Read the model definition and answer for the solid it produces. Units are mm, in the model's axes. A direction names the side the tool comes from. Coordinates: 2 decimals unless noted, no trailing zeros. Order: outer loops, then holes, each group sorted by start corner. A loop starts at its lowest first (then second) coordinate and runs counter-clockwise, first axis right, second up. Notation, with made-up numbers: (74.5, -27.5) -> (130.5, -27.5) arc R33 ccw to (130.5, 1.5) -> close; hole circle Ø5 at (60, 25). An arc over 180 degrees is marked (long way). Return JSON: item names as keys, results as strings. Group by question number.
```python
from build123d import *

# Parameters (mm, degrees)
F1_DEPTH  = 460
F3_D      = 6.5
F5_D      = 6.5
F7_D      = 6.5
F9_D      = 10.5
F9_DEPTH  = 3
F9_TIP    = 3.1545182499
F11_D     = 10.5
F11_DEPTH = 3
F11_TIP   = 3.1545182499
F13_D     = 10.5
F13_DEPTH = 3
F13_TIP   = 3.1545182499


with BuildPart() as f1:
    # F0 (on Front) → F1 (new body)
    with BuildSketch(Plane.XZ):
        Polygon((0, 10), (0, 0), (30, 0), (30, 5), (20, 5), (20, 10), align=None)
    extrude(amount=-F1_DEPTH)

    # F3 (through all)
    with Locations(Plane(origin=(0, 0, 0), x_dir=(1, 0, 0), z_dir=(0, 0, -1))):
        with Locations((10, -440)):
            Hole(F3_D / 2)

    # F5 (through all)
    with Locations(Plane(origin=(0, 0, 0), x_dir=(1, 0, 0), z_dir=(0, 0, -1))):
        with Locations((10, -230)):
            Hole(F5_D / 2)

    # F7 (through all)
    with Locations(Plane(origin=(0, 0, 0), x_dir=(1, 0, 0), z_dir=(0, 0, -1))):
        with Locations((10, -20)):
            Hole(F7_D / 2)

    # F9
    with Locations(Plane(origin=(0, 0, 0), x_dir=(1, 0, 0), z_dir=(0, 0, -1))):
        with Locations((10, -440)):
            Hole(F9_D / 2, depth=F9_DEPTH)
            with Locations((0, 0, -(F9_DEPTH + F9_TIP / 2))):  # 118° drill point
                Cone(0, F9_D / 2, F9_TIP, mode=Mode.SUBTRACT)

    # F11
    with Locations(Plane(origin=(0, 0, 0), x_dir=(1, 0, 0), z_dir=(0, 0, -1))):
        with Locations((10, -230)):
            Hole(F11_D / 2, depth=F11_DEPTH)
            with Locations((0, 0, -(F11_DEPTH + F11_TIP / 2))):  # 118° drill point
                Cone(0, F11_D / 2, F11_TIP, mode=Mode.SUBTRACT)

    # F13
    with Locations(Plane(origin=(0, 0, 0), x_dir=(1, 0, 0), z_dir=(0, 0, -1))):
        with Locations((10, -20)):
            Hole(F13_D / 2, depth=F13_DEPTH)
            with Locations((0, 0, -(F13_DEPTH + F13_TIP / 2))):  # 118° drill point
                Cone(0, F13_D / 2, F13_TIP, mode=Mode.SUBTRACT)


solid = f1.part
```
1. For a pull along X with two mould halves and no side action, classify faces 1 (the face through (0, 227, 5)), 2 (the face through (12, 227, 10)), 3 (the face through (5, 18.4, 1.5)) as released by +X, released by -X, zero draft, split by the parting line, or undercut.
2. Find section B-B on y = 323.5. Determine the outline of the cut face in (x, z), and give its area (3 significant figures).
3. Given pin 1 (5 mm diameter, centred on x = 10, y = 230, fed in from -Z); pin 2 (3 mm diameter, centred on x = 24.5, y = 162.5, fed in from +Z), each flat-ended and moving along its own axis, determine where each tip first touches the part or whether it passes through.
4. Find section A-A on z = 6.5. Determine the outline of the cut face in (x, y).
5. Straight lines are drawn through the part: L1, parallel to Y at x = 10, z = 7.2; L2, parallel to Y at x = 10, z = 1.6; L3, parallel to X at y = 20, z = 6.3. For each, find the intervals that lie inside material, in ascending order.
6. Which of the six approach directions +Z, -Z, +X, -X, +Y, -Y give full straight-line access (tool end or side, diameter ignored) to faces 4 (the face through (11, 0, 5)), 5 (the face through (7.18, 435.57, 1.52)), 6 (the face through (25, 227, 5))?
Result:
{
 "1": {"face 1": "released by -X", "face 2": "zero draft", "face 3": "undercut"},
 "2": {"outline": "(0, 0) -> (30, 0) -> (30, 5) -> (20, 5) -> (20, 10) -> (0, 10) -> close", "area": "250 mm^2"},
 "3": {"pin 1": "through", "pin 2": "z = 5"},
 "4": {"outline": "(0, 0) -> (20, 0) -> (20, 460) -> (0, 460) -> close; hole circle Ø6.5 at (10, 20); hole circle Ø6.5 at (10, 230); hole circle Ø6.5 at (10, 440)"},
 "5": {"L1": "0 to 16.75, 23.25 to 226.75, 233.25 to 436.75, 443.25 to 460", "L2": "0 to 14.75, 25.25 to 224.75, 235.25 to 434.75, 445.25 to 460", "L3": "0 to 6.75, 13.25 to 20"},
 "6": {"face 4": "+Z, -Z, +X, -X, -Y", "face 5": "-Z", "face 6": "+Z, +X, +Y, -Y"}
}
